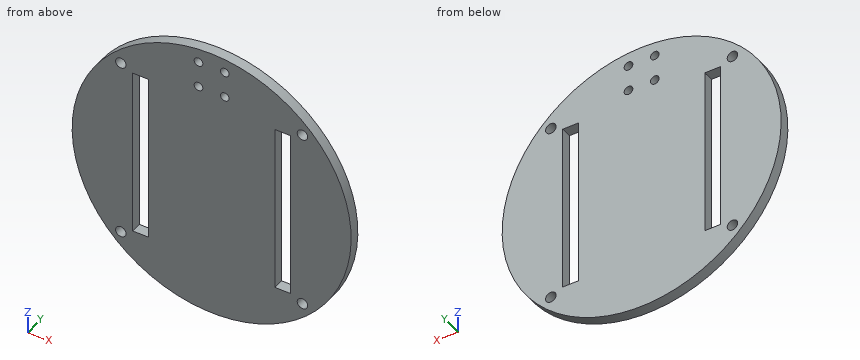
```python
from build123d import *

# Parameters (mm, degrees)
SKETCH1_R           = 84.1675
SKETCH1_W           = 9.525
SKETCH1_H           = 102.603301604
SKETCH1_R_2         = 2.6035
SKETCH1_R_3         = 3.175
BOSS_EXTRUDE1_DEPTH = 6.35


with BuildPart() as part:
    # Sketch1 → Boss-Extrude1 (new body)
    with BuildSketch(Plane(origin=(0, 66.8, 0), x_dir=(1, 0, 0), z_dir=(0, 1, 0))):
        with Locations(Location((0, 0, 0), (0, 0, 270))):
            Circle(SKETCH1_R)
        with Locations((-42.8625, 0)):
            Rectangle(SKETCH1_W, SKETCH1_H, mode=Mode.SUBTRACT)
        with Locations((42.8625, 0)):
            Rectangle(SKETCH1_W, SKETCH1_H, mode=Mode.SUBTRACT)
        with Locations(Location((-7.9375, -59.556650802, 0), (0, 0, 270))):
            Circle(SKETCH1_R_2, mode=Mode.SUBTRACT)
        with Locations(Location((7.9375, -59.556650802, 0), (0, 0, 270))):
            Circle(SKETCH1_R_2, mode=Mode.SUBTRACT)
        with Locations(Location((-54.800775542, -54.800775542, 0), (0, 0, 270))):
            Circle(SKETCH1_R_3, mode=Mode.SUBTRACT)
        with Locations(Location((-7.9375, -75.431650802, 0), (0, 0, 270))):
            Circle(SKETCH1_R_2, mode=Mode.SUBTRACT)
        with Locations(Location((7.9375, -75.431650802, 0), (0, 0, 270))):
            Circle(SKETCH1_R_2, mode=Mode.SUBTRACT)
        with Locations(Location((54.800775542, -54.800775542, 0), (0, 0, 270))):
            Circle(SKETCH1_R_3, mode=Mode.SUBTRACT)
        with Locations(Location((-54.800775542, 54.800775542, 0), (0, 0, 270))):
            Circle(SKETCH1_R_3, mode=Mode.SUBTRACT)
        with Locations(Location((54.800775542, 54.800775542, 0), (0, 0, 270))):
            Circle(SKETCH1_R_3, mode=Mode.SUBTRACT)
    extrude(amount=BOSS_EXTRUDE1_DEPTH)


solid = part.part
```
Input: part model. Units: mm. Frame: model coordinates. Round coordinates to 2 decimals unless told otherwise and drop trailing zeros. Loops run counter-clockwise (first coordinate to the right, second up) from the corner with the lowest first, then second, coordinate; pieces in that order, holes last. Notation, with made-up numbers: M 89,68 L 99,68 A30 cw 99,102 Z; hole C 38,84 d1. An arc over 180 degrees is marked long. Answer in a Markdown table with one row per item. Add a question column.
1. Section A-A (z = 0). Give the number of separate pieces and of enclosed holes in the cut face, and give its area (3 significant figures).
2. Ray query, probe 1 along X at (y, z) = (72, -36) (3 decimals); probe 2 along X at (y, z) = (69.5, 55); probe 3 along Z at (x, y) = (55.5, 71). Return the intervals inside material, ascending.
3. Section D-D (x = -70). Output: boundary loops of the cut face in (y, z), and give its area (3 significant figures).
4. Contact query for flat-ended pins moving along their axis: pin 1 (1 mm diameter, centred on x = -62, y = 71, fed in from -Z); pin 2 (3 mm diameter, centred on x = 45, y = 71, fed in from +Z); pin 3 (3 mm diameter, centred on y = 70.5, z = -10, fed in from -X). Output: stop coordinate, or through.
5. Section B-B (x = 44). Output: boundary loops of the cut face in (y, z), and give its area (3 significant figures).
Values follow:
| question | item | result |
|---|---|---|
| 1 | separate pieces | 3 |
| 1 | enclosed holes | 0 |
| 1 | area | 948 mm^2 |
| 2 | probe 1 | -76.08 to -47.625, -38.1 to 38.1, 47.625 to 76.08 |
| 2 | probe 2 | -63.71 to -57.97, -51.63 to 51.63, 57.97 to 63.71 |
| 2 | probe 3 | -63.28 to -57.9, -51.7 to 51.7, 57.9 to 63.28 |
| 3 | outline | M 66.8,-46.74 L 73.15,-46.74 L 73.15,46.74 L 66.8,46.74 Z |
| 3 | area | 594 mm^2 |
| 4 | pin 1 | z = -57.46 |
| 4 | pin 2 | z = 72.05 |
| 4 | pin 3 | x = -83.74 |
| 5 | outline | M 66.8,-71.75 L 73.15,-71.75 L 73.15,-51.3 L 66.8,-51.3 Z; M 66.8,51.3 L 73.15,51.3 L 73.15,71.75 L 66.8,71.75 Z |
| 5 | area | 260 mm^2 |
